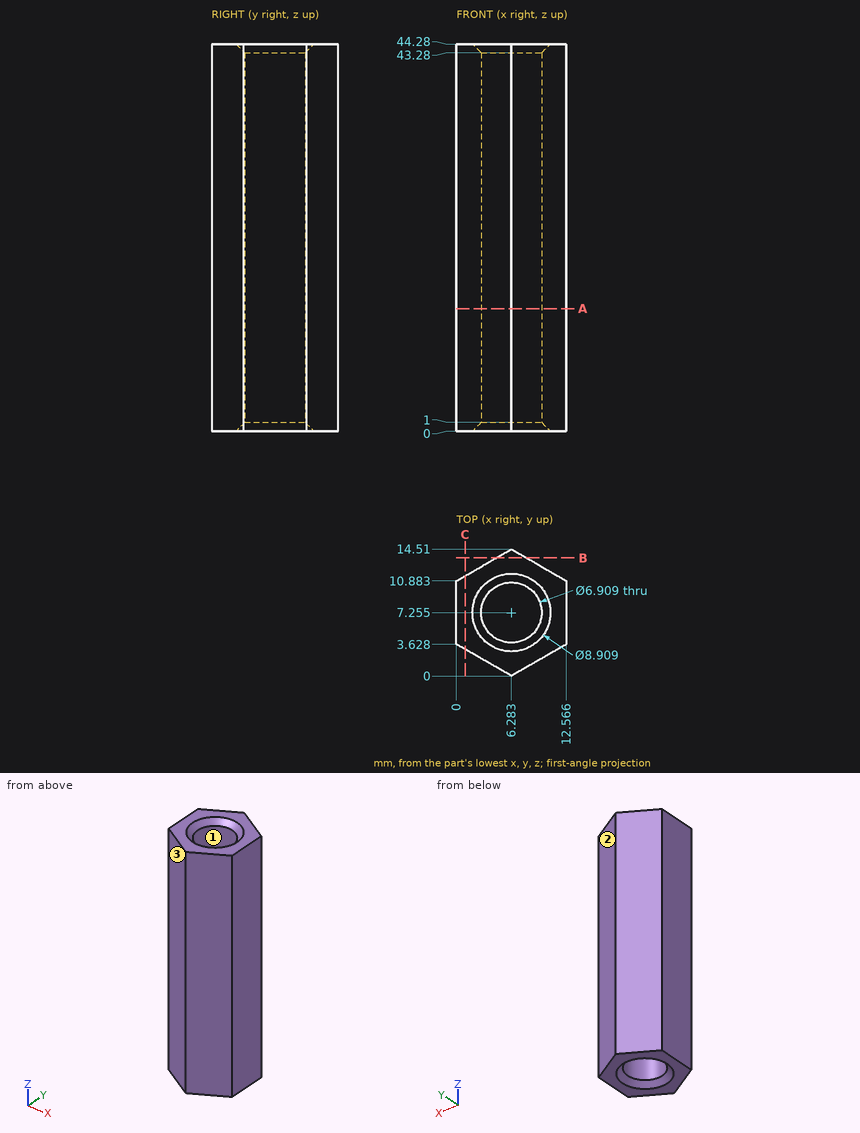
Study the drawing (mm; zero at the part's minimum x, y, z) and answer. Give positions to 0.01 mm unless a question says otherwise; leave off trailing zeros. Loops run counter-clockwise (first coordinate to the right, second up) from the corner with the lowest first, then second, coordinate; pieces in that order, holes last. Notation, with made-up numbers: (17.5, 86.25) - (63.5, 86.25) arc R21 cw to (63.5, 103.25) - close; hole circle Ø4 at (88.5, -25). An arc over 180 degrees is marked (long way). Answer in a Markdown table with one row per item. Add a question column.
Q1. The part is cut by section A-A (z = 14). Determine the outline of the cut face in (x, y) (1 decimal).
Q2. Consider line 1 along Y through (x, z) = (4.5, 41) (1 decimal); line 2 along X through (y, z) = (6.5, 29) (1 decimal); line 3 along Y through (x, z) = (7, 26) (1 decimal). Determine where each line is inside the solid, lowest interval first.
Q3. Each of these flat-tipped pins is pushed along its axis until it touches: P1, Ø6, axis at x = 3, z = 18, coming from the -Y side; P2, Ø6, axis at x = 5.5, z = 34, coming from the +Y side; P3, Ø2, axis at x = 9.5, z = 6.5, coming from the +Y side. Where does it stop, or does it pass through?
Q4. The part is cut by section B-B (y = 13.5). Determine the outline of the cut face in (x, z), and give its area (3 significant figures).
Q5. Determine the mould class of the marked faces 1, 2 and 3 for opening direction X: released by +X, released by -X, zero draft, split by the parting line, or undercut.
Q6. The part is cut by section C-C (x = 1). Determine the outline of the cut face in (y, z).
Solution:
| question | item | result |
|---|---|---|
| 1 | outline | (0, 3.6) - (6.3, 0) - (12.6, 3.6) - (12.6, 10.9) - (6.3, 14.5) - (0, 10.9) - close; hole circle Ø6.9 at (6.3, 7.3) |
| 2 | line 1 | y = 1 to 4.3, 10.2 to 13.5 |
| 2 | line 2 | x = 0 to 2.9, 9.7 to 12.6 |
| 2 | line 3 | y = 0.4 to 3.9, 10.6 to 14.1 |
| 3 | P1 | stops at y = 0.16 |
| 3 | P2 | stops at y = 14.51 |
| 3 | P3 | stops at y = 13.23 |
| 4 | outline | (4.53, 0) - (8.03, 0) - (8.03, 44.28) - (4.53, 44.28) - close |
| 4 | area | 155 mm² |
| 5 | face 1 | undercut |
| 5 | face 2 | released by +X |
| 5 | face 3 | released by -X |
| 6 | outline | (3.05, 0) - (11.46, 0) - (11.46, 44.28) - (3.05, 44.28) - close |
